The model under review builds one solid part; all positions refer to its coordinate system, in mm. A direction names the side the tool comes from. Round coordinates to 2 decimals unless told otherwise and drop trailing zeros. Write each loop counter-clockwise with the first axis right and the second up, starting at its lowest first coordinate (ties: lowest second). Pieces come first, ordered by that corner, then holes. Notation, with made-up numbers: (-13.5, -18) -> (13.5, -18) arc R22 ccw to (13.5, 6) -> close; hole circle Ø5 at (24.25, 21.25). An arc over 180 degrees is marked (long way). Return JSON: item names as keys, results as strings. Group by question number.
1. Take a section at B-B, the plane x = 0. Write out the cut boundary in (y, z) (1 decimal).
2. For line 1 along X through (y, z) = (1, 2.35); line 2 along Y through (x, z) = (-3.25, 1.8); line 3 along Y through (x, z) = (-2.25, 0.8), list the stretches that pass through material, from the lowest coordinate up. Write a range as from..to.
3. Mouldability with a two-part tool opening along Y and no side actions: class faces 3 (the flat face through (4, -4, 0)), 4 (the flat face through (0, -4.762, 2)), 5 (the cylindrical face through (-1.323, 10.074, 1.579)) as pulls with the +Y half, pulls with the -Y half, needs draft (parallel to the pull), parting line crosses it, or undercut.
4. Tool access review of faces 1 (the flat face through (-4.11, 2.41, 1.57)), 2 (the flat face through (4, -4, 3.175)): name each direction out of +Z, -Z, +X, -X, +Y, -Y from which nothing blocks a thin tool from reaching the whole face with its end or side.
5. Clearance check with flat-ended pins moving along their axes: P1, Ø1, axis at y = 1.5, z = 3, coming from the -X side; P2, Ø2, axis at x = -5, y = 5, coming from the -Z side; P3, Ø1.6, axis at x = 1, z = 2.5, coming from the +Y side; P4, Ø1.5, axis at y = 3, z = 0.5, coming from the -X side. State where each tip first meets the part, or that it passes through.
6. Take a section at A-A, the plane z = 1.4. Write out the cut boundary in (x, y).
from build123d import *

# Parameters (mm, degrees)
SKETCH1_R           = 10.16
BOSS_EXTRUDE1_DEPTH = 3.175
CHAMFER1_SIZE       = 1


with BuildPart() as part:
    # Sketch1 → Boss-Extrude1 (new body)
    with BuildSketch(Plane.XY):
        Circle(SKETCH1_R)
        Polygon((5.499261314, 0), (2.749630657, 4.7625), (-2.749630657, 4.7625), (-5.499261314, 0), (-2.749630657, -4.7625), (2.749630657, -4.7625), align=None, mode=Mode.SUBTRACT)
    extrude(amount=BOSS_EXTRUDE1_DEPTH)

    # Chamfer1
    chamfer1_edges = [part.edges().sort_by_distance(p)[0] for p in [
        (-10.16, 0, 0),
        (-10.16, 0, 3.175),
    ]]
    chamfer(chamfer1_edges, length=CHAMFER1_SIZE)


solid = part.part
Output:
{
 "1": {"outline": "(-10.2, 1) -> (-9.2, 0) -> (-4.8, 0) -> (-4.8, 3.2) -> (-9.2, 3.2) -> (-10.2, 2.2) -> close; (4.8, 0) -> (9.2, 0) -> (10.2, 1) -> (10.2, 2.2) -> (9.2, 3.2) -> (4.8, 3.2) -> close"},
 "2": {"line 1": "x = -9.93..-4.92, 4.92..9.93", "line 2": "y = -9.63..-3.9, 3.9..9.63", "line 3": "y = -9.7..-4.76, 4.76..9.7"},
 "3": {"face 3": "needs draft", "face 4": "undercut", "face 5": "parting line crosses it"},
 "4": {"face 1": "+Z, -Z", "face 2": "+Z, +X, -X, +Y, -Y"},
 "5": {"P1": "stops at x = -9.73", "P2": "stops at z = 0", "P3": "stops at y = 10.16", "P4": "stops at x = -9.86"},
 "6": {"outline": "circle Ø20.32 at (0, 0); hole (-5.5, 0) -> (-2.75, -4.76) -> (2.75, -4.76) -> (5.5, 0) -> (2.75, 4.76) -> (-2.75, 4.76) -> close"}
}
